Autodesk Inventor part; units mm, degrees
ref_plane "YZ Plane" through (0, 0, 0) normal (1, 0, 0) x (0, 1, 0)
ref_plane "XZ Plane" through (0, 0, 0) normal (0, 1, 0) x (-1, 0, 0)
ref_plane "XY Plane" through (0, 0, 0) normal (0, 0, 1) x (1, 0, 0)
sketch "Sketch1" plane through (0, 0, 0) normal (0, 0, 1) x (1, 0, 0)
  circle A0 centre (0, 0) radius 2.5
  circle A1 centre (0, 0) radius 4.5
  circle A2 centre (0, -9) radius 1.25
  circle A3 centre (0, -9) radius 3
  circle A4 centre (0, -9) radius 4
  circle A5 centre (0, 0) radius 1.25
  line L0 (-4.4931, -0.25) -> (-3.9938, -9.2222)
  line L1 (4.4931, -0.25) -> (3.9938, -9.2222)
  line L2 (0, 0) -> (0, -19.0302) construction
  point P0 (66.1895, -52.0583)
  point P1 (148.6808, -39.1685)
  point P2 (99.1548, -7.9801)
  point P3 (101.772, -8.3287)
  point P4 (96.5376, -8.3287)
  dimension "d8" = 9
  dimension "d13" = 5
  dimension "d25" = 2.5
  dimension "d26" = 6
  dimension "d27" = 8
  dimension "d28" = 2.5
  dimension "d29" = 9
extrude "Extrusion1" add sketch "Sketch1" along normal blind 0.5 contours A1 | A1 L1 A4 L0 | A4
extrude "Extrusion2" add sketch "Sketch1" along normal blind 2 contours A0 | A3
properties part number "ヘッケン抑え"
Verification items for the finished model (mm, model axes). A direction names the side the tool comes from. Give positions to 0.01 mm unless a question says otherwise; leave off trailing zeros. Order: outer loops, then holes, each group sorted by start corner. A loop starts at its lowest first (then second) coordinate and runs counter-clockwise, first axis right, second up. Notation, with made-up numbers: (-5.5, 17) -> (29.5, 17) arc R17 ccw to (29.5, 41) -> close; hole circle Ø4 at (20.25, 39.25). An arc over 180 degrees is marked (long way). Use a Markdown table: item, result.
1) Section check B-B, the plane y = 0. Record the boundary of the cut face in (x, z), then the cut area to 3 significant figures.
Results:
| item | result |
|---|---|
| outline | (-4.5, 0) -> (-1.25, 0) -> (-1.25, 2) -> (-2.5, 2) -> (-2.5, 0.5) -> (-4.5, 0.5) -> close; (1.25, 0) -> (4.5, 0) -> (4.5, 0.5) -> (2.5, 0.5) -> (2.5, 2) -> (1.25, 2) -> close |
| area | 7.00 mm² |
2) Section check D-D, the plane y = -9. Record the boundary of the cut face in (x, z), then the cut area to 3 significant figures.
Results:
| item | result |
|---|---|
| outline | (-4.01, 0) -> (-1.25, 0) -> (-1.25, 2) -> (-3, 2) -> (-3, 0.5) -> (-4.01, 0.5) -> close; (1.25, 0) -> (4.01, 0) -> (4.01, 0.5) -> (3, 0.5) -> (3, 2) -> (1.25, 2) -> close |
| area | 8.01 mm² |
3) Material ranges on probe 1 along Y at (x, z) = (0, 1.2); probe 2 along Y at (x, z) = (-1, 0.6); probe 3 along Z at (x, y) = (0.5, -12), recorded low to high.
Results:
| item | result |
|---|---|
| probe 1 | -12 to -10.25, -7.75 to -6, -2.5 to -1.25, 1.25 to 2.5 |
| probe 2 | -11.83 to -9.75, -8.25 to -6.17, -2.29 to -0.75, 0.75 to 2.29 |
| probe 3 | 0 to 0.5 |
4) Section check C-C, the plane z = 1.7. Record the boundary of the cut face in (x, y).
Results:
| item | result |
|---|---|
| outline | circle Ø6 at (0, -9); circle Ø5 at (0, 0); hole circle Ø2.5 at (0, -9); hole circle Ø2.5 at (0, 0) |
5) Tool access check on faces 4 (the flat face through (0, -4, 0)), 5 (the cylindrical face through (-3, -9, 1)). Record the directions out of +Z, -Z, +X, -X, +Y, -Y that give a thin tool (end or side, any length) a straight path to the whole face; none if there is none.
Results:
| item | result |
|---|---|
| face 4 | -Z, +X, -X, +Y, -Y |
| face 5 | +Z |
6) Section check A-A, the plane x = 0. Record the boundary of the cut face in (y, z).
Results:
| item | result |
|---|---|
| outline | (-13, 0) -> (-10.25, 0) -> (-10.25, 2) -> (-12, 2) -> (-12, 0.5) -> (-13, 0.5) -> close; (-7.75, 0) -> (-1.25, 0) -> (-1.25, 2) -> (-2.5, 2) -> (-2.5, 0.5) -> (-6, 0.5) -> (-6, 2) -> (-7.75, 2) -> close; (1.25, 0) -> (4.5, 0) -> (4.5, 0.5) -> (2.5, 0.5) -> (2.5, 2) -> (1.25, 2) -> close |
7) Mould release check, pull along X, two halves, no side actions. Record for faces 1 (the flat face through (1, 1, 2)), 2 (the cylindrical face through (-0.16, -10.24, 0.99)), 3 (the cylindrical face through (-0.1, 4.5, 0.2)): pulls with the +X half, pulls with the -X half, needs draft (parallel to the pull), parting line crosses it, or undercut.
Results:
| item | result |
|---|---|
| face 1 | needs draft |
| face 2 | undercut |
| face 3 | parting line crosses it |
8) Depth check by flat-ended pin: pin 1 Ø1 at (x, z) = (-1, 1.5) entering from +Y; pin 2 Ø1.5 at (x, y) = (0, -9) entering from +Z. Enter the tip coordinate at first touch or a pass-through.
Results:
| item | result |
|---|---|
| pin 1 | y = 2.45 |
| pin 2 | through |
